Source: CAD feature listing. Evaluate the final solid. Frame: model axes, mm. Round coordinates to 2 decimals unless told otherwise and drop trailing zeros. Loops run counter-clockwise (first coordinate to the right, second up) from the corner with the lowest first, then second, coordinate; pieces in that order, holes last. Notation, with made-up numbers: M 21.25,11.5 L 68.25,11.5 A24 ccw 68.25,21.5 Z; hole C 73,60.5 d2. An arc over 180 degrees is marked long. Answer as a JSON object with one key per item and string values.
from build123d import *

# Parameters (mm, degrees)
SKETCH_1_W          = 105
SKETCH_1_H          = 53.5
EXTRUDE_1_DEPTH     = 3
SKETCH_2_R          = 1.55
SKETCH_2_W          = 2
SKETCH_2_H          = 12
CUT_EXTRUDE_1_DEPTH = 5
SKETCH_3_W          = 7
SKETCH_3_H          = 26
SKETCH_3_W_2        = 12
CUT_EXTRUDE_2_DEPTH = 4
SKETCH_8_W          = 105
SKETCH_8_H          = 2.5
EXTRUDE_2_DEPTH     = 3
FILLET_1_R          = 2
SKETCH_7_R          = 0.5
CUT_EXTRUDE_6_DEPTH = 10
SKETCH_10_W         = 0.05
SKETCH_10_H         = 12
EXTRUDE_3_DEPTH     = 3
SKETCH_11_R         = 0.5
CUT_EXTRUDE_7_DEPTH = 10
SKETCH_12_R         = 2.05
CUT_EXTRUDE_8_DEPTH = 10


with BuildPart() as part:
    # 草图1 → 凸台-拉伸1 (new body)
    with BuildSketch(Plane.XY):
        Rectangle(SKETCH_1_W, SKETCH_1_H)
    extrude(amount=EXTRUDE_1_DEPTH)

    # 草图2 → 切除-拉伸1 (cut)
    with BuildSketch(Plane(origin=(0, 0, 0), x_dir=(-1, 0, 0), z_dir=(0, 0, -1))):
        with Locations((46, -9.25)):
            Circle(SKETCH_2_R)
        with Locations((-46, -9.25)):
            Circle(SKETCH_2_R)
        with Locations((42.5, -18.25)):
            Rectangle(SKETCH_2_W, SKETCH_2_H)
        with Locations((-42.5, -18.25)):
            Rectangle(SKETCH_2_W, SKETCH_2_H)
    extrude(amount=-CUT_EXTRUDE_1_DEPTH, mode=Mode.SUBTRACT)

    # 草图3 → 切除-拉伸2 (cut, through all)
    with BuildSketch(Plane(origin=(0, 0, 0), x_dir=(-1, 0, 0), z_dir=(0, 0, -1))):
        with Locations((-28, 13.75)):
            Rectangle(SKETCH_3_W, SKETCH_3_H)
        with Locations((-14, 13.75)):
            Rectangle(SKETCH_3_W, SKETCH_3_H)
        with Locations((46.5, 13.75)):
            Rectangle(SKETCH_3_W_2, SKETCH_3_H)
        with Locations((28, 13.75)):
            Rectangle(SKETCH_3_W, SKETCH_3_H)
        with Locations((0, 13.75)):
            Rectangle(SKETCH_3_W, SKETCH_3_H)
        with Locations((-46.5, 13.75)):
            Rectangle(SKETCH_3_W_2, SKETCH_3_H)
        with Locations((14, 13.75)):
            Rectangle(SKETCH_3_W, SKETCH_3_H)
    extrude(amount=-CUT_EXTRUDE_2_DEPTH, mode=Mode.SUBTRACT)

    # 草图8 → 凸台-拉伸2 (add)
    with BuildSketch(Plane(origin=(0, 0, 0), x_dir=(-1, 0, 0), z_dir=(0, 0, -1))):
        with Locations((0, -28)):
            Rectangle(SKETCH_8_W, SKETCH_8_H)
    extrude(amount=-EXTRUDE_2_DEPTH)

    # 圆角1
    fillet_1_edges = [part.edges().sort_by_distance(p)[0] for p in [
        (-52.5, 0.75, 1.5),
        (52.5, 0.75, 1.5),
        (-52.5, -29.25, 1.5),
        (52.5, -29.25, 1.5),
    ]]
    fillet(fillet_1_edges, radius=FILLET_1_R)

    # 草图7 → 切除-拉伸6 (cut)
    with BuildSketch(Plane(origin=(0, 0, 0), x_dir=(-1, 0, 0), z_dir=(0, 0, -1))):
        with Locations((-40.5, 0.75)):
            Circle(SKETCH_7_R)
        with Locations((-31.5, 0.75)):
            Circle(SKETCH_7_R)
        with Locations((-24.5, 0.75)):
            Circle(SKETCH_7_R)
        with Locations((-17.5, 0.75)):
            Circle(SKETCH_7_R)
        with Locations((-10.5, 0.75)):
            Circle(SKETCH_7_R)
        with Locations((24.5, 0.75)):
            Circle(SKETCH_7_R)
        with Locations((31.5, 0.75)):
            Circle(SKETCH_7_R)
        with Locations((40.5, 0.75)):
            Circle(SKETCH_7_R)
        with Locations((-3.5, 0.75)):
            Circle(SKETCH_7_R)
        with Locations((3.5, 0.75)):
            Circle(SKETCH_7_R)
        with Locations((10.5, 0.75)):
            Circle(SKETCH_7_R)
        with Locations((17.5, 0.75)):
            Circle(SKETCH_7_R)
    extrude(amount=-CUT_EXTRUDE_6_DEPTH, mode=Mode.SUBTRACT)

    # 草图10 → 凸台-拉伸3 (add)
    with BuildSketch(Plane(origin=(0, 0, 0), x_dir=(-1, 0, 0), z_dir=(0, 0, -1))):
        with Locations((43.475, -18.25)):
            Rectangle(SKETCH_10_W, SKETCH_10_H)
        with Locations((41.525, -18.25)):
            Rectangle(SKETCH_10_W, SKETCH_10_H)
        with Locations((-41.525, -18.25)):
            Rectangle(SKETCH_10_W, SKETCH_10_H)
        with Locations((-43.475, -18.25)):
            Rectangle(SKETCH_10_W, SKETCH_10_H)
    extrude(amount=-EXTRUDE_3_DEPTH)

    # 草图11 → 切除-拉伸7 (cut)
    with BuildSketch(Plane(origin=(0, 0, 0), x_dir=(-1, 0, 0), z_dir=(0, 0, -1))):
        with Locations((43.45, -24.25)):
            Circle(SKETCH_11_R)
        with Locations((41.55, -24.25)):
            Circle(SKETCH_11_R)
        with Locations((43.45, -12.25)):
            Circle(SKETCH_11_R)
        with Locations((41.55, -12.25)):
            Circle(SKETCH_11_R)
        with Locations((-41.55, -24.25)):
            Circle(SKETCH_11_R)
        with Locations((-43.45, -24.25)):
            Circle(SKETCH_11_R)
        with Locations((-43.45, -12.25)):
            Circle(SKETCH_11_R)
        with Locations((-41.55, -12.25)):
            Circle(SKETCH_11_R)
    extrude(amount=-CUT_EXTRUDE_7_DEPTH, mode=Mode.SUBTRACT)

    # 草图12 → 切除-拉伸8 (cut)
    with BuildSketch(Plane(origin=(0, 0, 0), x_dir=(-1, 0, 0), z_dir=(0, 0, -1))):
        with Locations((-30.5, -4.25)):
            Circle(SKETCH_12_R)
        with Locations((-20.5, -4.25)):
            Circle(SKETCH_12_R)
        with Locations((20.5, -4.25)):
            Circle(SKETCH_12_R)
        with Locations((30.5, -4.25)):
            Circle(SKETCH_12_R)
    extrude(amount=-CUT_EXTRUDE_8_DEPTH, mode=Mode.SUBTRACT)


solid = part.part
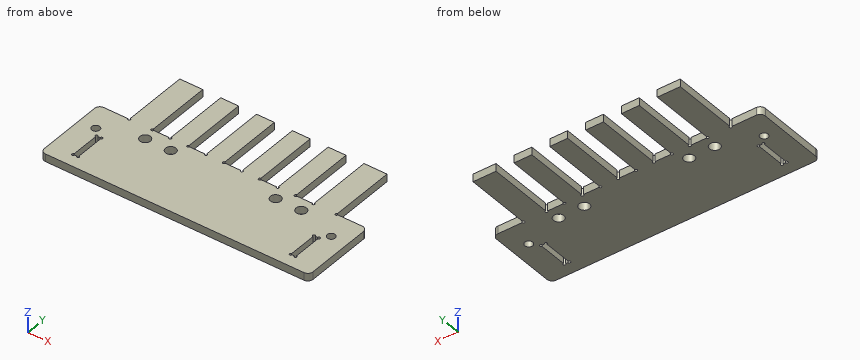
Item 1: Section D-D on x = -27. Return the cut outline in (y, z).
Answer sheet:
{"outline": "M -29.25,0 L 0.75,0 L 0.75,3 L -29.25,3 Z"}
Item 2: Line query: probe 1 along X at (y, z) = (8, 0.3); probe 2 along Y at (x, z) = (46, 2.1); probe 3 along X at (y, z) = (-23, 2.3). Output: solid intervals per line, ascending. Write a range as from..to.
Answer sheet:
{"probe 1": "x = -40.5..-31.5, -24.5..-17.5, -10.5..-3.5, 3.5..10.5, 17.5..24.5, 31.5..40.5", "probe 2": "y = -29.25..-10.8, -7.7..0.75", "probe 3": "x = -52.5..-43.45, -41.55..41.55, 43.45..52.5"}
Item 3: Section A-A on y = 9.5. Return the cut outline in (x, z), then the cut area to 3 significant figures.
Answer sheet:
{"outline": "M -40.5,0 L -31.5,0 L -31.5,3 L -40.5,3 Z; M -24.5,0 L -17.5,0 L -17.5,3 L -24.5,3 Z; M -10.5,0 L -3.5,0 L -3.5,3 L -10.5,3 Z; M 3.5,0 L 10.5,0 L 10.5,3 L 3.5,3 Z; M 17.5,0 L 24.5,0 L 24.5,3 L 17.5,3 Z; M 31.5,0 L 40.5,0 L 40.5,3 L 31.5,3 Z", "area": "138 mm²"}
Item 4: Section C-C on z = 2.3. Give the number of separate pieces and of enclosed holes in the cut face, then the cut area to 3 significant figures.
Answer sheet:
{"separate pieces": "1", "enclosed holes": "8", "area": "4,220 mm²"}
Item 5: Contact query for flat-ended pins moving along their axis: pin 1 Ø1.5 at (y, z) = (11, 1.5) entering from +X; pin 2 Ø1.5 at (y, z) = (19.5, 2) entering from -X; pin 3 Ø0.9 at (x, z) = (46, 1) entering from +Y. Output: stop coordinate, or through.
Answer sheet:
{"pin 1": "stops at x = 40.5", "pin 2": "stops at x = -40.5", "pin 3": "stops at y = 0.75"}
Item 6: Section B-B on y = -16.5. Return the cut outline in (x, z), then the cut area to 3 significant figures.
Answer sheet:
{"outline": "M -52.5,0 L -43.45,0 L -43.45,3 L -52.5,3 Z; M -41.55,0 L 41.55,0 L 41.55,3 L -41.55,3 Z; M 43.45,0 L 52.5,0 L 52.5,3 L 43.45,3 Z", "area": "304 mm²"}
